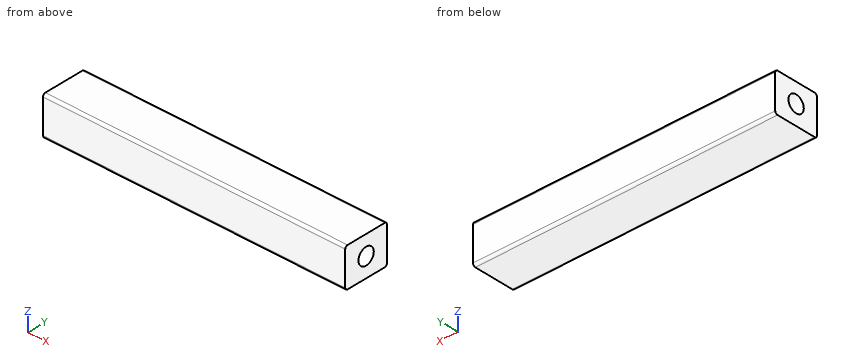
from build123d import *

# Parameters (mm, degrees)
SKETCH1_W           = 15.5
SKETCH1_H           = 18
BOSS_EXTRUDE1_DEPTH = 60
FILLET1_R           = 1


with BuildPart() as part:
    # Sketch1 → Boss-Extrude1 (new body, symmetric)
    with BuildSketch(Plane(origin=(0, 0, 0), x_dir=(0, 0, -1), z_dir=(1, 0, 0))):
        Rectangle(SKETCH1_W, SKETCH1_H)
    extrude(amount=BOSS_EXTRUDE1_DEPTH, both=True)

    # Fillet1
    fillet1_edges = [part.edges().sort_by_distance(p)[0] for p in [
        (0, -9, -7.75),
        (0, -9, 7.75),
        (0, 9, 7.75),
        (0, 9, -7.75),
    ]]
    fillet(fillet1_edges, radius=FILLET1_R)

    # Sketch3 → Ø1.0 (6.6) Diameter Hole1 (revolve, cut)
    with BuildSketch(Plane(origin=(60, 0, 0), x_dir=(0, 0, -1), z_dir=(0, 1, 0))):
        Polygon((0, 0), (0, 13.982840043), (3.3, 12), (3.3, 0), align=None)
    f_1_0_6_6_diameter_hole1 = revolve(axis=Axis((66.35, 0, 0), (-1, 0, 0)), mode=Mode.SUBTRACT)

    # Mirror1: Ø1.0 (6.6) Diameter Hole1 across plane
    add(f_1_0_6_6_diameter_hole1.mirror(Plane(origin=(0, 0, 0), x_dir=(0, 0, 1), z_dir=(1, 0, 0))), mode=Mode.SUBTRACT)


solid = part.part
Can you work these out from the model? Positions are in its coordinate system, mm. Round coordinates to 2 decimals unless told otherwise and drop trailing zeros. Loops run counter-clockwise (first coordinate to the right, second up) from the corner with the lowest first, then second, coordinate; pieces in that order, holes last. Notation, with made-up numbers: (-5, 53) - (7, 53) arc R7 cw to (7, 63) - close; hole circle Ø4 at (-19, 10.5). An arc over 180 degrees is marked (long way). Write item = value, one per line. Start each with the question number.
(1) For P1, Ø4, axis at y = 0, z = 0, coming from the +X side, with a flat end and sliding along its axis, tell me the tip position at first contact or that it passes through.
(2) If we section it at A-A (x = 47): Please give me the cut outline in (y, z), and give its area (3 significant figures).
(3) If I drill on probe 1 along Y at (x, z) = (-50.75, 0); probe 2 along Z at (x, y) = (54, 0); probe 3 along Y at (x, z) = (-55, 2.5), over which ranges is the centre line in solid material (lowest first)? Write a range as [from, to].
Ans:
q1.P1 = 47.22
q2.outline = (-9, -6.75) arc R1 ccw to (-8, -7.75) - (8, -7.75) arc R1 ccw to (9, -6.75) - (9, 6.75) arc R1 ccw to (8, 7.75) - (-8, 7.75) arc R1 ccw to (-9, 6.75) - close; hole circle Ø3.27 at (0, 0)
q2.area = 270 mm²
q3.probe_1 = [-9, -3.3], [3.3, 9]
q3.probe_2 = [-7.75, -3.3], [3.3, 7.75]
q3.probe_3 = [-9, -2.15], [2.15, 9]
